from build123d import *

# Parameters (mm, degrees)
BOSS_EXTRUDE3_OUTLINE_R = 3
BOSS_EXTRUDE3_DEPTH     = 102
CUT_EXTRUDE1_DEPTH      = 102
CUT_EXTRUDE2_DEPTH      = 102
SKETCH4_W               = 0.4
SKETCH4_H               = 1.8
SKETCH4_W_2             = 1.8
SKETCH4_H_2             = 0.4
BOSS_EXTRUDE4_DEPTH     = 102
SKETCH5_W               = 75
SKETCH5_H               = 43.392810524
CUT_EXTRUDE6_DEPTH      = 10
SKETCH7_R               = 3.05
CUT_EXTRUDE9_DEPTH      = 147.084376475


# Read off the part's stored shape, not the designer's step: Boss-Extrude3
with BuildPart() as part:
    # Boss-Extrude3 outline → Boss-Extrude3 (new body)
    with BuildSketch(Plane.XY):
        with BuildLine():
            add(Edge.make_bspline(
                [(24.392810524, -72.348554199), (27.040667073, -69.541086329), (29.089162938, -67.428574969), (30.241441862, -64.355831171), (31.073643307, -60.963009895), (30.561519341, -59.042545022), (29.217193929, -56.673971678), (27.488775543, -54.241382838), (25.105954954, -53), (17.37432721, -53), (-19, -52.782560411)],
                knots=[0, 0, 0, 0, 0, 0, 0, 0, 0, 0, 0, 1, 1, 1, 1, 1, 1, 1, 1, 1, 1, 1], degree=10))
            ThreePointArc((24.392810524, -72.348554199), (55.939709188, -51.962211615), (73.948106805, -19))
            Line((73.948106805, -19), (52.782560411, -19))
            add(Edge.make_bspline(
                [(72.348554199, 24.392810524), (69.541086329, 27.040667073), (67.428574969, 29.089162938), (64.355831171, 30.241441862), (60.963009895, 31.073643307), (59.042545022, 30.561519341), (56.673971678, 29.217193929), (54.241382838, 27.488775543), (53, 25.105954954), (53, 17.37432721), (52.782560411, -19)],
                knots=[0, 0, 0, 0, 0, 0, 0, 0, 0, 0, 0, 1, 1, 1, 1, 1, 1, 1, 1, 1, 1, 1], degree=10))
            ThreePointArc((72.348554199, 24.392810524), (51.962211615, 55.939709188), (19, 73.948106805))
            Line((19, 73.948106805), (19, 53))
            add(Edge.make_bspline(
                [(-24.392810524, 72.348554199), (-27.040667073, 69.541086329), (-29.089162938, 67.428574969), (-30.241441862, 64.355831171), (-31.073643307, 60.963009895), (-30.561519341, 59.042545022), (-29.217193929, 56.673971678), (-27.488775543, 54.241382838), (-25.105954954, 53), (-17.37432721, 53), (19, 53)],
                knots=[0, 0, 0, 0, 0, 0, 0, 0, 0, 0, 0, 1, 1, 1, 1, 1, 1, 1, 1, 1, 1, 1], degree=10))
            ThreePointArc((-24.392810524, 72.348554199), (-55.939709188, 51.962211615), (-73.948106805, 19))
            Line((-73.948106805, 19), (-52.782560411, 19))
            add(Edge.make_bspline(
                [(-72.348554199, -24.392810524), (-69.541086329, -27.040667073), (-67.428574969, -29.089162938), (-64.355831171, -30.241441862), (-60.963009895, -31.073643307), (-59.042545022, -30.561519341), (-56.673971678, -29.217193929), (-54.241382838, -27.488775543), (-53, -25.105954954), (-53, -17.37432721), (-52.782560411, 19)],
                knots=[0, 0, 0, 0, 0, 0, 0, 0, 0, 0, 0, 1, 1, 1, 1, 1, 1, 1, 1, 1, 1, 1], degree=10))
            ThreePointArc((-72.348554199, -24.392810524), (-51.962211615, -55.939709188), (-19, -73.948106805))
            Line((-19, -73.948106805), (-19, -52.782560411))
        make_face()
        with Locations((-30, -58.782560411)):
            Circle(BOSS_EXTRUDE3_OUTLINE_R, mode=Mode.SUBTRACT)
        with Locations((58.782560411, -30)):
            Circle(BOSS_EXTRUDE3_OUTLINE_R, mode=Mode.SUBTRACT)
        with Locations((-58.782560411, 30)):
            Circle(BOSS_EXTRUDE3_OUTLINE_R, mode=Mode.SUBTRACT)
        Polygon((-38.9, -51.6), (-51.6, -51.6), (-51.6, -38.9), (-50, -38.9), (-50, 38.9), (-51.6, 38.9), (-51.6, 51.6), (-38.9, 51.6), (-38.9, 50), (38.9, 50), (38.9, 51.6), (51.6, 51.6), (51.6, 38.9), (50, 38.9), (50, -38.9), (51.6, -38.9), (51.6, -51.6), (38.9, -51.6), (38.9, -50), (-38.9, -50), align=None, mode=Mode.SUBTRACT)
        with Locations((30, 59)):
            Circle(BOSS_EXTRUDE3_OUTLINE_R, mode=Mode.SUBTRACT)
    extrude(amount=BOSS_EXTRUDE3_DEPTH)

    # Sketch2 → Cut-Extrude1 (cut)
    with BuildSketch(Plane.XY.offset(102)):
        Polygon((51.8, -38.7), (50.2, -38.7), (50.2, 38.7), (51.8, 38.7), (51.8, 51.8), (38.7, 51.8), (38.7, 50.2), (-38.7, 50.2), (-38.7, 51.8), (-51.8, 51.8), (-51.8, 38.7), (-50.2, 38.7), (-50.2, -38.7), (-51.8, -38.7), (-51.8, -51.8), (-38.7, -51.8), (-38.7, -50.2), (38.7, -50.2), (38.7, -51.8), (51.8, -51.8), align=None)
        Polygon((51.6, -38.9), (50, -38.9), (50, 38.9), (51.6, 38.9), (51.6, 51.6), (38.9, 51.6), (38.9, 50), (-38.9, 50), (-38.9, 51.6), (-51.6, 51.6), (-51.6, 38.9), (-50, 38.9), (-50, -38.9), (-51.6, -38.9), (-51.6, -51.6), (-38.9, -51.6), (-38.9, -50), (38.9, -50), (38.9, -51.6), (51.6, -51.6), align=None, mode=Mode.SUBTRACT)
    extrude(amount=-CUT_EXTRUDE1_DEPTH, mode=Mode.SUBTRACT)

    # Sketch3 → Cut-Extrude2 (cut)
    with BuildSketch(Plane.XY.offset(102)):
        Polygon((-51.8, -51.8), (-38.7, -51.8), (-38.7, -52), (-52, -52), (-52, -38.7), (-51.8, -38.7), align=None)
        Polygon((38.7, -51.8), (51.8, -51.8), (51.8, -38.7), (52, -38.7), (52, -52), (38.7, -52), align=None)
        Polygon((51.8, 38.7), (51.8, 51.8), (38.7, 51.8), (38.7, 52), (52, 52), (52, 38.7), align=None)
        Polygon((-51.8, 51.8), (-51.8, 38.7), (-52, 38.7), (-52, 52), (-38.7, 52), (-38.7, 51.8), align=None)
    extrude(amount=-CUT_EXTRUDE2_DEPTH, mode=Mode.SUBTRACT)

    # Sketch4 → Boss-Extrude4 (add)
    with BuildSketch(Plane.XY.offset(102)):
        with Locations((-38.9, 51.1)):
            Rectangle(SKETCH4_W, SKETCH4_H)
        with Locations((-51.1, 38.9)):
            Rectangle(SKETCH4_W_2, SKETCH4_H_2)
        with Locations((38.9, 51.1)):
            Rectangle(SKETCH4_W, SKETCH4_H)
        with Locations((51.1, 38.9)):
            Rectangle(SKETCH4_W_2, SKETCH4_H_2)
        with Locations((38.9, -51.1)):
            Rectangle(SKETCH4_W, SKETCH4_H)
        with Locations((51.1, -38.9)):
            Rectangle(SKETCH4_W_2, SKETCH4_H_2)
        with Locations((-51.1, -38.9)):
            Rectangle(SKETCH4_W_2, SKETCH4_H_2)
        with Locations((-38.9, -51.1)):
            Rectangle(SKETCH4_W, SKETCH4_H)
    extrude(amount=-BOSS_EXTRUDE4_DEPTH)

    # Sketch5 → Cut-Extrude6 (cut)
    with BuildSketch(Plane.ZY.offset(-50.2)):
        with Locations((49, 2.696405262)):
            Rectangle(SKETCH5_W, SKETCH5_H)
    extrude(amount=-CUT_EXTRUDE6_DEPTH, mode=Mode.SUBTRACT)

    # Sketch7 → Cut-Extrude9 (cut, through all)
    with BuildSketch(Plane(origin=(0, 0, 0), x_dir=(-1, 0, 0), z_dir=(0, 0, -1))):
        with Locations((30, -58.782560411)):
            Circle(SKETCH7_R)
        with Locations((-58.782560411, -30)):
            Circle(SKETCH7_R)
        with Locations((58.782560411, 30)):
            Circle(SKETCH7_R)
        with Locations((-30, 59)):
            Circle(SKETCH7_R)
    extrude(amount=-CUT_EXTRUDE9_DEPTH, mode=Mode.SUBTRACT)


solid = part.part
Design review of the part built by this model. Coordinates are the model's own, in mm. A direction names the side the tool comes from. Coordinates: 2 decimals unless noted, no trailing zeros. Put each result on its own line as item: value.
1) Insertion check: P1, Ø1.5, axis at x = 39.5, z = 18.5, coming from the -Y side; P2, Ø1.5, axis at x = -37, z = 32.5, coming from the -Y side; P3, Ø10.5, axis at y = -66.5, z = 64, coming from the +X side; P4, Ø8, axis at x = -58.78, y = 30, coming from the +Z side. Each pin has a flat end and moves straight along its axis. Give the tip position at first contact, or say it passes through.
Response values:
P1: stops at y = -65.79
P2: stops at y = -67.2
P3: stops at x = 45.58
P4: stops at z = 102
2) Take a section at A-A, the plane y = 4. Count the separate pieces of the cut face and the enclosed holes in it, and give its area (3 significant figures).
Response values:
separate pieces: 3
enclosed holes: 0
area: 349 mm²
3) Tool access review of faces 1 (the face through (46, -52, 52)), 2 (the face through (-19, -64, 50)), 3 (the face through (-55.577, 52.35, 50.286)): name each direction out of +Z, -Z, +X, -X, +Y, -Y from which nothing blocks a thin tool from reaching the whole face with its end or side.
Response values:
face 1: +Z, -Z
face 2: +Z, -Z, -Y
face 3: +Z, -Z, -X, +Y
4) The part is to be moulded in two halves that separate along Y. For faces 4 (the face through (54, -22, 102)), 5 (the face through (52, -45, 52)), 6 (the face through (-52.35, -55.577, 50.286)), say which applies: released by +Y, released by -Y, zero draft, split by the parting line, or undercut.
Response values:
face 4: zero draft
face 5: undercut
face 6: released by -Y
5) Wall thickness on L1, parallel to X at y = 31, z = 46.5; L2, parallel to Y at x = 30, z = 38; L3, parallel to Y at x = 32.5, z = 54.5: over which ranges is each line inside the solid? List them lowest first. Write a range as from..to.
Response values:
L1: x = -69.77..-61.66, -55.9..-50.2, 50.2..69.77
L2: y = -70.21..-50.2, 50.2..55.95, 62.05..70.21
L3: y = -69.09..-50.2, 50.2..57.25, 60.75..69.09
